For this review, use the dimensioned drawing (mm, ordinates from the lowest corner) and the shaded views. A direction names the side the tool comes from. Give positions to 0.01 mm unless a question says otherwise; leave off trailing zeros. Loops run counter-clockwise (first coordinate to the right, second up) from the corner with the lowest first, then second, coordinate; pieces in that order, holes last. Notation, with made-up numbers: M 60.25,67.5 L 90.25,67.5 A29 cw 90.25,97.5 Z; hole C 48.5,37 d5. An arc over 180 degrees is marked long. Use CSV: the item, a comma, the result in double quotes.
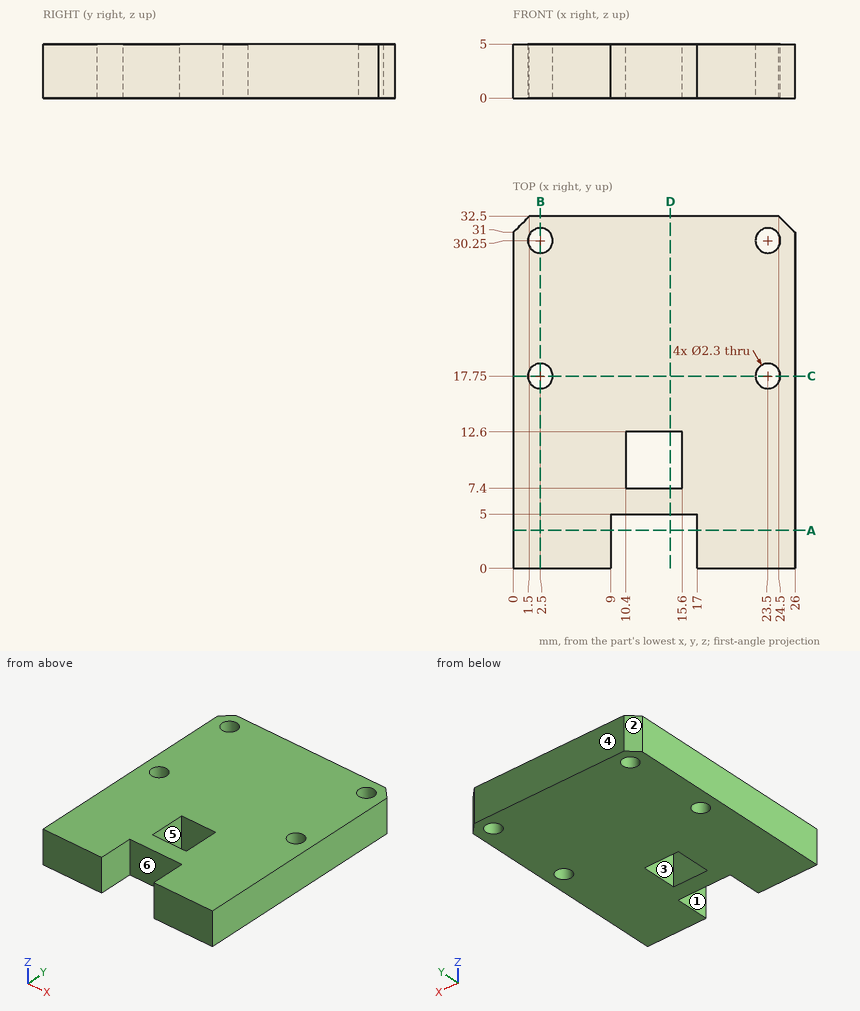
(1) We need section A-A on y = 3.5. State the section outline as (x, z) points.
A:
outline,"M 0,0 L 9,0 L 9,5 L 0,5 Z; M 17,0 L 26,0 L 26,5 L 17,5 Z"
(2) We need section D-D on x = 14.5. State the section outline as (y, z) points, then the cut area to 4 significant figures.
A:
outline,"M 5,0 L 7.4,0 L 7.4,5 L 5,5 Z; M 12.6,0 L 32.5,0 L 32.5,5 L 12.6,5 Z"
area,"111.5 mm²"
(3) We need section B-B on x = 2.5. State the section outline as (y, z) points.
A:
outline,"M 0,0 L 16.6,0 L 16.6,5 L 0,5 Z; M 18.9,0 L 29.1,0 L 29.1,5 L 18.9,5 Z; M 31.4,0 L 32.5,0 L 32.5,5 L 31.4,5 Z"
(4) Machinability: for the marked faces 4, 5 and 6, which of the approach directions +Z, -Z, +X, -X, +Y, -Y give a long, thin tool a straight path to every point of the face, cutting with its end or side? Answer none if there is none.
A:
face 4,"+Z, -Z, +X, -X, +Y"
face 5,"+Z, -Z"
face 6,"+Z, -Z, -Y"
(5) Wall thickness on line 1 along Y through (x, z) = (23.5, 2.5); line 2 along Y through (x, z) = (13.5, 4.4); line 3 along Y through (x, z) = (3.25, 2.85): over which ranges is each line inside the solid? List them lowest first. Write a range as [from, to].
A:
line 1,"[0, 16.6], [18.9, 29.1], [31.4, 32.5]"
line 2,"[5, 7.4], [12.6, 32.5]"
line 3,"[0, 16.88], [18.62, 29.38], [31.12, 32.5]"
(6) The part is to be moulded in two halves that separate along Y. For the marked faces 1, 2 and 3, say which applies: released by +Y, released by -Y, zero draft, split by the parting line, or undercut.
A:
face 1,"zero draft"
face 2,"released by +Y"
face 3,"undercut"
(7) We need section C-C on y = 17.75. State the section outline as (x, z) points.
A:
outline,"M 0,0 L 1.35,0 L 1.35,5 L 0,5 Z; M 3.65,0 L 22.35,0 L 22.35,5 L 3.65,5 Z; M 24.65,0 L 26,0 L 26,5 L 24.65,5 Z"
